Source: CAD feature listing. Evaluate the final solid. Frame: model axes, mm. Give positions to 0.01 mm unless a question says otherwise; leave off trailing zeros. Loops run counter-clockwise (first coordinate to the right, second up) from the corner with the lowest first, then second, coordinate; pieces in that order, holes last. Notation, with made-up numbers: M -20.5,43 L 13.5,43 A15 ccw 13.5,58 Z; hole C 20,58.25 d5. An arc over 180 degrees is marked long. Put each result on its own line as item: value. Start each with the question number.
```python
from build123d import *

# Parameters (mm, degrees)
SKETCH1_R           = 40
BOSS_EXTRUDE1_DEPTH = 100
SKETCH2_R           = 15
CUT_EXTRUDE1_DEPTH  = 5
BOSS_EXTRUDE2_DEPTH = 5
SKETCH4_R           = 2.5
CUT_EXTRUDE2_DEPTH  = 5


with BuildPart() as part:
    # Sketch1 → Boss-Extrude1 (new body)
    with BuildSketch(Plane(origin=(0, 0, 0), x_dir=(1, 0, 0), z_dir=(0, 1, 0))):
        Circle(SKETCH1_R)
        with BuildLine():
            Line((-2.5, 34.910600109), (-2.5, -34.910600109))
            ThreePointArc((-2.5, -34.910600109), (-35, 0), (-2.5, 34.910600109))
        make_face(mode=Mode.SUBTRACT)
        with BuildLine():
            Line((2.5, 34.910600109), (2.5, -34.910600109))
            ThreePointArc((2.5, -34.910600109), (35, 0), (2.5, 34.910600109))
        make_face(mode=Mode.SUBTRACT)
    extrude(amount=-BOSS_EXTRUDE1_DEPTH)

    # Sketch2 → Cut-Extrude1 (cut)
    with BuildSketch(Plane(origin=(2.5, 0, 0), x_dir=(0, 0, -1), z_dir=(1, 0, 0))):
        with Locations((0, -75)):
            Circle(SKETCH2_R)
    extrude(amount=-CUT_EXTRUDE1_DEPTH, mode=Mode.SUBTRACT)

    # Sketch3 → Revolve1 (revolve)
    with BuildSketch(Plane(origin=(0, 0, 0), x_dir=(0, 0, -1), z_dir=(1, 0, 0))):
        with BuildLine():
            Line((35, -100), (40, -100))
            ThreePointArc((40, -100), (28.284271247, -128.284271247), (0, -140))
            Line((0, -140), (0, -135))
            ThreePointArc((0, -135), (24.748737342, -124.748737342), (35, -100))
        make_face()
    revolve1 = revolve(axis=Axis((0, -140, 0), (0, 1, 0)))

    # Sketch1_2 → Boss-Extrude2 (add)
    with BuildSketch(Plane(origin=(0, 0, 0), x_dir=(1, 0, 0), z_dir=(0, 1, 0))):
        with BuildLine():
            Line((-2.5, 34.910600109), (-2.5, -34.910600109))
            ThreePointArc((-2.5, -34.910600109), (-35, 0), (-2.5, 34.910600109))
        make_face()
        with BuildLine():
            ThreePointArc((2.5, 34.910600109), (35, 0), (2.5, -34.910600109))
            Line((2.5, -34.910600109), (2.5, 34.910600109))
        make_face()
    extrude(amount=-BOSS_EXTRUDE2_DEPTH)

    # Sketch4 → Cut-Extrude2 (cut)
    with BuildSketch(Plane(origin=(0, 0, 0), x_dir=(1, 0, 0), z_dir=(0, 1, 0))):
        with Locations((-15, 0)):
            Circle(SKETCH4_R)
        with Locations((15, 0)):
            Circle(SKETCH4_R)
    extrude(amount=-CUT_EXTRUDE2_DEPTH, mode=Mode.SUBTRACT)

    # Mirror1: Revolve1 across plane
    add(revolve1.mirror(Plane.ZX.offset(-50)))


solid = part.part
```
1. Ray query, line 1 (X direction, y = -3.45, z = 0); line 2 (Y direction, x = -18, z = 12.5); line 3 (Y direction, x = -29, z = -7.5). Return the intervals inside material, ascending.
2. Section A-A, the plane z = 0. Output: boundary loops of the cut face in (x, y).
3. Contact query for flat-ended pins moving along their axis: pin 1 (9.5 mm diameter, centred on x = 25.5, z = 1.5, fed in from -Y); pin 2 (6 mm diameter, centred on y = 16.5, z = 9.5, fed in from -X); pin 3 (9.5 mm diameter, centred on x = -25.5, z = 5.5, fed in from -Y). Output: stop coordinate, or through.
4. Section C-C, the plane y = -75. Output: boundary loops of the cut face in (x, z), plus the area to 3 significant figures.
5. Section B-B, the plane x = 0. Output: boundary loops of the cut face in (y, z), plus the area to 3 significant figures.
6. Pull-direction query (Y, two-part tool) for faces 1 (the face through (-17.5, -2.5, -0.1)), 2 (the face through (-8.67, -49.3, 39.05)); classes: released by +Y, released by -Y, zero draft, split by the parting line, or undercut.
7. Section D-D, the plane x = -31.5. Output: boundary loops of the cut face in (y, z), plus the area to 3 significant figures.
Results found:
1. line 1: -40 to -17.5, -12.5 to 12.5, 17.5 to 40
1. line 2: -133.46 to -127.29, -5 to 0, 27.29 to 33.46
1. line 3: -126.51 to -118.1, -5 to 0, 18.1 to 26.51
2. outline: M -40,-100 A40 ccw 40,-100 L 40,0 A40 ccw -40,0 Z; M -12.5,-5 L -2.5,-5 L -2.5,-60 L 2.5,-60 L 2.5,-5 L 12.5,-5 L 12.5,0 L -12.5,0 Z; M -2.5,-100 L 2.5,-100 L 2.5,-90 L -2.5,-90 Z; hole M -35,-100 A35 ccw 35,-100 L 35,-5 L 17.5,-5 L 17.5,0 L 35,0 A35 ccw -35,0 L -17.5,0 L -17.5,-5 L -35,-5 Z
3. pin 1: y = -134.17
3. pin 2: x = -36.64
3. pin 3: y = -133.83
4. outline: C 0,0 d80; hole M -2.5,-34.91 L -2.5,-15 L 2.5,-15 L 2.5,-34.91 A35 ccw 2.5,34.91 L 2.5,15 L -2.5,15 L -2.5,34.91 A35 ccw Z
4. area: 1,380 mm²
5. outline: M -100,-40 L 0,-40 A40 ccw 0,40 L -100,40 A40 ccw Z; hole M -100,-35 L -100,35 A35 ccw Z; hole C -75,0 d30; hole M 0,-35 A35 ccw 0,35 Z
5. area: 8,470 mm²
6. face 1: undercut
6. face 2: zero draft
7. outline: M -100,-24.65 L 0,-24.65 A24.65 ccw 0,24.65 L -100,24.65 A24.65 ccw Z; hole M -100,-15.26 L -5,-15.26 L -5,15.26 L -100,15.26 A15.26 ccw Z; hole M 0,-15.26 A15.26 ccw 0,15.26 Z
7. area: 3,210 mm²
